Design review of the part built by this model. Coordinates are the model's own, in mm. A direction names the side the tool comes from. Round coordinates to 2 decimals unless told otherwise and drop trailing zeros. Order: outer loops, then holes, each group sorted by start corner. A loop starts at its lowest first (then second) coordinate and runs counter-clockwise, first axis right, second up.
from build123d import *

# Parameters (mm, degrees)
ESBO_O1_W                = 119
ESBO_O1_H                = 44
RESSALTO_EXTRUS_O2_DEPTH = 2
ESBO_O2_W                = 119
ESBO_O2_H                = 44
ESBO_O2_W_2              = 115
ESBO_O2_H_2              = 40
RESSALTO_EXTRUS_O3_DEPTH = 35
RESSALTO_EXTRUS_O5_DEPTH = 3
ESBO_O5_W                = 3
ESBO_O5_H                = 40
RESSALTO_EXTRUS_O6_DEPTH = 7
ESBO_O8_W                = 9
ESBO_O8_H                = 4
CORTE_EXTRUS_O1_DEPTH    = 7
ESBO_O9_W                = 17
ESBO_O9_H                = 13
CORTE_EXTRUS_O2_DEPTH    = 7
CORTE_EXTRUS_O5_DEPTH    = 7
RESSALTO_EXTRUS_O7_DEPTH = 3
ESPELHAR3_COPY_1_DEPTH   = 3
ESPELHAR3_COPY_2_DEPTH   = 3
ESBO_O12_W               = 3
ESBO_O12_H               = 3
CORTE_EXTRUS_O6_DEPTH    = 6
ESBO_O13_W               = 6.5
ESBO_O13_H               = 3.5
CORTE_EXTRUS_O7_DEPTH    = 10


with BuildPart() as part:
    # Esboço1 → Ressalto-extrusão2 (new body)
    with BuildSketch(Plane(origin=(0, 0, 0), x_dir=(1, 0, 0), z_dir=(0, 1, 0))):
        Rectangle(ESBO_O1_W, ESBO_O1_H)
    extrude(amount=RESSALTO_EXTRUS_O2_DEPTH)

    # Esboço2 → Ressalto-extrusão3 (add)
    with BuildSketch(Plane(origin=(0, 2, 0), x_dir=(1, 0, 0), z_dir=(0, 1, 0))):
        Rectangle(ESBO_O2_W, ESBO_O2_H)
        Rectangle(ESBO_O2_W_2, ESBO_O2_H_2, mode=Mode.SUBTRACT)
    extrude(amount=RESSALTO_EXTRUS_O3_DEPTH)

    # Esboço3 → Ressalto-extrusão5 (add)
    with BuildSketch(Plane(origin=(0, 2, 0), x_dir=(1, 0, 0), z_dir=(0, 1, 0))):
        Polygon((-57.5, -15), (-57.5, -20), (-14.5, -20), (-14.5, -1), (-57.5, -1), (-57.5, -6), (-46.5, -6), (-46.5, -15), align=None)
        Polygon((-14.5, -1), (-14.5, -20), (-11.5, -20), (-11.5, 20), (-14.5, 20), align=None)
    extrude(amount=RESSALTO_EXTRUS_O5_DEPTH)

    # Esboço5 → Ressalto-extrusão6 (add)
    with BuildSketch(Plane(origin=(0, 5, 0), x_dir=(1, 0, 0), z_dir=(0, 1, 0))):
        with Locations((-13, 0)):
            Rectangle(ESBO_O5_W, ESBO_O5_H)
    extrude(amount=RESSALTO_EXTRUS_O6_DEPTH)

    # Esboço8 → Corte-extrusão1 (cut)
    with BuildSketch(Plane(origin=(-57.5, 0, 0), x_dir=(0, 0, -1), z_dir=(1, 0, 0))):
        with Locations((-10.5, 4)):
            Rectangle(ESBO_O8_W, ESBO_O8_H)
    extrude(amount=-CORTE_EXTRUS_O1_DEPTH, mode=Mode.SUBTRACT)

    # Esboço9 → Corte-extrusão2 (cut)
    with BuildSketch(Plane(origin=(-57.5, 0, 0), x_dir=(0, 0, -1), z_dir=(1, 0, 0))):
        with Locations((9.5, 8.5)):
            Rectangle(ESBO_O9_W, ESBO_O9_H)
    extrude(amount=-CORTE_EXTRUS_O2_DEPTH, mode=Mode.SUBTRACT)

    # Esboço10 → Corte-extrusão5 (cut)
    with BuildSketch(Plane(origin=(59.5, 0, 0), x_dir=(0, 0, -1), z_dir=(1, 0, 0))):
        Polygon((-16, 26), (16, 26), (16, 28), (18, 28), (18, 32), (16, 32), (16, 34), (-16, 34), (-16, 32), (-18, 32), (-18, 28), (-16, 28), align=None)
    extrude(amount=-CORTE_EXTRUS_O5_DEPTH, mode=Mode.SUBTRACT)

    # Esboço11 → Ressalto-extrusão7 (add)
    with BuildSketch(Plane(origin=(0, 37, 0), x_dir=(1, 0, 0), z_dir=(0, 1, 0))):
        Polygon((-59.5, 22), (-59.5, 12), (-49.5, 22), align=None)
    ressalto_extrus_o7 = extrude(amount=-RESSALTO_EXTRUS_O7_DEPTH)

    # Espelhar1: Ressalto-extrusão7 across plane
    add(ressalto_extrus_o7.mirror(Plane.XY))

    # Espelhar2: Ressalto-extrusão7 across plane
    add(ressalto_extrus_o7.mirror(Plane(origin=(0, 0, 0), x_dir=(0, 0, 1), z_dir=(1, 0, 0))))

    # Espelhar3 copy 1 sketch → Espelhar3 copy 1 (add)
    with BuildSketch(Plane(origin=(0, 37, 0), x_dir=(-1, 0, 0), z_dir=(0, 1, 0))):
        Polygon((-59.5, 22), (-59.5, 12), (-49.5, 22), align=None)
    extrude(amount=-ESPELHAR3_COPY_1_DEPTH)

    # Espelhar3 copy 2 sketch → Espelhar3 copy 2 (add)
    with BuildSketch(Plane(origin=(0, 37, 0), x_dir=(-1, 0, 0), z_dir=(0, 1, 0))):
        Polygon((-59.5, -22), (-59.5, -12), (-49.5, -22), align=None)
    extrude(amount=-ESPELHAR3_COPY_2_DEPTH)

    # Esboço12 → Corte-extrusão6 (cut)
    with BuildSketch(Plane(origin=(0, 12, 0), x_dir=(1, 0, 0), z_dir=(0, 1, 0))):
        with Locations((-13, 0.25)):
            Rectangle(ESBO_O12_W, ESBO_O12_H)
    extrude(amount=-CORTE_EXTRUS_O6_DEPTH, mode=Mode.SUBTRACT)

    # Esboço13 → Corte-extrusão7 (cut)
    with BuildSketch(Plane.ZY.offset(59.5)):
        with Locations((10.25, 25.155612263)):
            Rectangle(ESBO_O13_W, ESBO_O13_H)
    extrude(amount=-CORTE_EXTRUS_O7_DEPTH, mode=Mode.SUBTRACT)


solid = part.part
1) Take a section at C-C on x = -0.5. Give the boundary of the cut face in (y, z).
Results:
outline: (0, -22) - (37, -22) - (37, -20) - (2, -20) - (2, 20) - (37, 20) - (37, 22) - (0, 22) - close
2) For faces 4 (the face through (59, 28, 17)), 5 (the face through (-59, 26.906, 10)), 6 (the face through (-58, 6, 11)), 7 (the face through (-54.5, 35.5, -17)), 8 (the face through (57.5, 14, 0)), list the 3-axis set-ups (+Z, -Z, +X, -X, +Y, -Y) from which the entire face can be reached by the end or side of a thin tool; tool diameter is ignored.
Results:
face 4: +X
face 5: +X, -X
face 6: -X
face 7: +Y
face 8: none
3) Take a section at A-A on z = 3.5. Give the boundary of the cut face in (x, y).
Results:
outline: (-59.5, 0) - (59.5, 0) - (59.5, 26) - (57.5, 26) - (57.5, 2) - (-11.5, 2) - (-11.5, 12) - (-14.5, 12) - (-14.5, 5) - (-57.5, 5) - (-57.5, 37) - (-59.5, 37) - close; (57.5, 34) - (59.5, 34) - (59.5, 37) - (57.5, 37) - close
4) The part is to be moulded in two halves that separate along Y. For faces 1 (the face through (-53, 4, 15)), 2 (the face through (-59.5, 18, 0)), 3 (the face through (-13, 12, 10)), say which applies: released by +Y, released by -Y, zero draft, split by the parting line, or undercut.
Results:
face 1: undercut
face 2: zero draft
face 3: released by +Y
5) Take a section at B-B on z = -10. Give the boundary of the cut face in (x, y).
Results:
outline: (-59.5, 0) - (59.5, 0) - (59.5, 26) - (57.5, 26) - (57.5, 2) - (-11.5, 2) - (-11.5, 12) - (-14.5, 12) - (-14.5, 2) - (-59.5, 2) - close; (-59.5, 15) - (-57.5, 15) - (-57.5, 37) - (-59.5, 37) - close; (57.5, 34) - (59.5, 34) - (59.5, 37) - (57.5, 37) - close
6) To check wall thickness, follow line 1 along Z through (x, y) = (2, 3.5); line 2 along X through (y, z) = (35.5, -9.5); line 3 along X through (y, z) = (10.5, -10.5). State the ranges of each line that lie inside material, in increasing order.
Results:
line 1: z = -22 to -20, 20 to 22
line 2: x = -59.5 to -57.5, 57.5 to 59.5
line 3: x = -14.5 to -11.5, 57.5 to 59.5
7) Take a section at D-D on y = 21. Give the boundary of the cut face in (x, z).
Results:
outline: (-59.5, -22) - (59.5, -22) - (59.5, 22) - (-59.5, 22) - close; hole (-57.5, -20) - (57.5, -20) - (57.5, 20) - (-57.5, 20) - close
8) Clearance check with flat-ended pins moving along their axes: P1, Ø1.5, axis at x = 26, z = -1.5, coming from the +Y side; P2, Ø0.9, axis at x = -13.5, z = 0, coming from the +Y side. State where each tip first meets the part, or that it passes through.
Results:
P1: stops at y = 2
P2: stops at y = 6
